Could you check a few things on this model? Use its own coordinates, in mm. A direction names the side the tool comes from. Give positions to 0.01 mm unless a question says otherwise; leave off trailing zeros. Order: outer loops, then holes, each group sorted by start corner. A loop starts at its lowest first (then second) coordinate and runs counter-clockwise, first axis right, second up. Notation, with made-up numbers: (66.5, 28) -> (121.5, 28) arc R25 ccw to (121.5, 41) -> close; hole circle Ø7 at (-21.75, 57). An arc over 180 degrees is marked (long way). Answer as CSV lines item,"result". Start each with the question number.
(1) I want a section at C-C (z = 0.55). Please give me the cut outline in (x, y) (3 decimals), plus the area to 3 significant figures.
(2) On a 3-axis mill with a long thin cutter (end or side, diameter ignored), from which of +Z, -Z, +X, -X, +Y, -Y can I reach the whole of each face in a straight line? I mean faces 1 (the face through (0, -5, 0)), 2 (the face through (3.175, -11, 1)). Say none if no direction works.
(3) I want a section at D-D (x = -9). Please give me the cut outline in (y, z) (3 decimals), plus the area to 3 significant figures.
(4) Will these pins go through, and if not, where does the flat tip stop? pin 1 Ø1.3 at (y, z) = (10, 1) entering from -X; pin 2 Ø0.8 at (x, z) = (-13.5, 1.5) entering from -Y; pin 3 Ø0.8 at (x, z) = (13, 1.5) entering from -Y.
(5) We'd pull the mould along X, two halves only. Please class faces 3 (the face through (0, -5, 2.54)), 4 (the face through (13.59, 13.35, 1.25)), 5 (the face through (-5.506, -24.796, 1.252)): released by +X, released by -X, zero draft, split by the parting line, or undercut.
(6) I need wall thicknesses on L1, parallel to Y at x = 0, z = 1.35 (3 decimals); L2, parallel to Y at x = -14.5, z = 2.1 (1 decimal); L3, parallel to X at y = 15, z = 1.2 (3 decimals). Which ranges of each line are inside material? Lowest first, please.
(7) I want a section at A-A (x = 0). Please give me the cut outline in (y, z) (3 decimals), plus the area to 3 significant figures.
```python
from build123d import *

# Parameters (mm, degrees)
SKETCH1_R           = 25.4
BOSS_EXTRUDE1_DEPTH = 2.54
SKETCH1_4_R         = 3.175
CUT_EXTRUDE2_DEPTH  = 2.54


with BuildPart() as part:
    # Sketch1 → Boss-Extrude1 (new body)
    with BuildSketch(Plane.XY):
        Circle(SKETCH1_R)
    extrude(amount=BOSS_EXTRUDE1_DEPTH)

    # Sketch1<4> → Cut-Extrude2 (cut)
    with BuildSketch(Plane.XY):
        with BuildLine():
            Line((-3.175, -18.783553311), (-3.175, -3.175))
            Line((-3.175, -3.175), (-18.783553311, -3.175))
            ThreePointArc((-18.783553311, -3.175), (-13.470384182, -13.470384182), (-3.175, -18.783553311))
        make_face()
        with BuildLine():
            Line((-18.783553311, 3.175), (-3.175, 3.175))
            Line((-3.175, 3.175), (-3.175, 18.783553311))
            ThreePointArc((-3.175, 18.783553311), (-13.470384182, 13.470384182), (-18.783553311, 3.175))
        make_face()
        with BuildLine():
            Line((3.175, 18.783553311), (3.175, 3.175))
            Line((3.175, 3.175), (18.783553311, 3.175))
            ThreePointArc((18.783553311, 3.175), (13.470384182, 13.470384182), (3.175, 18.783553311))
        make_face()
        with BuildLine():
            Line((18.783553311, -3.175), (3.175, -3.175))
            Line((3.175, -3.175), (3.175, -18.783553311))
            ThreePointArc((3.175, -18.783553311), (13.470384182, -13.470384182), (18.783553311, -3.175))
        make_face()
        Circle(SKETCH1_4_R)
    extrude(amount=CUT_EXTRUDE2_DEPTH, mode=Mode.SUBTRACT)


solid = part.part
```
Final values:
1,outline,"circle Ø50.8 at (0, 0); hole (-18.784, -3.175) arc R19.05 ccw to (-3.175, -18.784) -> (-3.175, -3.175) -> close; hole (-18.784, 3.175) -> (-3.175, 3.175) -> (-3.175, 18.784) arc R19.05 ccw to start; hole circle Ø6.35 at (0, 0); hole (3.175, -18.784) arc R19.05 ccw to (18.784, -3.175) -> (3.175, -3.175) -> close; hole (3.175, 3.175) -> (18.784, 3.175) arc R19.05 ccw to (3.175, 18.784) -> close"
1,area,"1,300 mm²"
2,face 1,"-Z, +X, -X, +Y, -Y"
2,face 2,"+Z, -Z"
3,outline,"(-23.752, 0) -> (-16.79, 0) -> (-16.79, 2.54) -> (-23.752, 2.54) -> close; (-3.175, 0) -> (3.175, 0) -> (3.175, 2.54) -> (-3.175, 2.54) -> close; (16.79, 0) -> (23.752, 0) -> (23.752, 2.54) -> (16.79, 2.54) -> close"
3,area,"51.5 mm²"
4,pin 1,"x = -23.62"
4,pin 2,"y = -21.76"
4,pin 3,"y = -22.05"
5,face 3,"zero draft"
5,face 4,"undercut"
5,face 5,"split by the parting line"
6,L1,"-25.4 to -3.175, 3.175 to 25.4"
6,L2,"-20.9 to -12.4, -3.2 to 3.2, 12.4 to 20.9"
6,L3,"-20.498 to -11.743, -3.175 to 3.175, 11.743 to 20.498"
7,outline,"(-25.4, 0) -> (-3.175, 0) -> (-3.175, 2.54) -> (-25.4, 2.54) -> close; (3.175, 0) -> (25.4, 0) -> (25.4, 2.54) -> (3.175, 2.54) -> close"
7,area,"113 mm²"
